```python
from build123d import *

# Parameters (mm, degrees)
BOSS_EXTRUDE1_DEPTH = 20
BOSS_EXTRUDE2_DEPTH = 20
SKETCH4_R           = 5
CUT_EXTRUDE1_DEPTH  = 2
SKETCH5_R           = 7
CUT_EXTRUDE2_DEPTH  = 2
BOSS_EXTRUDE5_DEPTH = 5
BOSS_EXTRUDE6_DEPTH = 2
SKETCH11_W          = 20
SKETCH11_H          = 5
SKETCH12_W          = 5
SKETCH12_H          = 5
BOSS_EXTRUDE7_DEPTH = 5
SKETCH13_R          = 1.5
BOSS_EXTRUDE8_DEPTH = 5
FILLET1_R           = 2.5


with BuildPart() as part:
    # Sketch2 → Boss-Extrude1 (new body)
    with BuildSketch(Plane(origin=(0, 0, 0), x_dir=(0, 0, -1), z_dir=(1, 0, 0))):
        with BuildLine():
            Line((-50, 0), (-45, 0))
            ThreePointArc((-45, 0), (0, 45), (45, 0))
            Line((45, 0), (50, 0))
            ThreePointArc((50, 0), (0, 50), (-50, 0))
        make_face()
    extrude(amount=BOSS_EXTRUDE1_DEPTH)

    # Sketch3 → Boss-Extrude2 (add)
    with BuildSketch(Plane(origin=(0, 0, 0), x_dir=(0, 0, -1), z_dir=(1, 0, 0))):
        Polygon((0, 45), (8, 45), (8, 50), (-8, 50), (-8, 45), align=None)
    extrude(amount=BOSS_EXTRUDE2_DEPTH)

    # Sketch4 → Cut-Extrude1 (cut)
    with BuildSketch(Plane(origin=(0, 50, 0), x_dir=(1, 0, 0), z_dir=(0, 1, 0))):
        with Locations(Location((10, 0, 0), (0, 0, 270))):
            Circle(SKETCH4_R)
    extrude(amount=-CUT_EXTRUDE1_DEPTH, mode=Mode.SUBTRACT)

    # Sketch5 → Cut-Extrude2 (cut)
    with BuildSketch(Plane(origin=(0, 48, 0), x_dir=(1, 0, 0), z_dir=(0, 1, 0))):
        with Locations(Location((10, 0, 0), (0, 0, 270))):
            Circle(SKETCH5_R)
    extrude(amount=-CUT_EXTRUDE2_DEPTH, mode=Mode.SUBTRACT)

    # Sketch9 → Boss-Extrude5 (add)
    with BuildSketch(Plane.ZY):
        with BuildLine():
            Line((10, 46.946778377), (11.041666667, 51.837067792))
            ThreePointArc((11.041666667, 51.837067792), (5.551369518, 52.708465131), (0, 53))
            Line((0, 53), (0, 48))
            ThreePointArc((0, 48), (5.027655412, 47.735968421), (10, 46.946778377))
        make_face()
    extrude(amount=BOSS_EXTRUDE5_DEPTH)

    # Sketch10 → Boss-Extrude6 (add)
    with BuildSketch(Plane.ZY.offset(5)):
        with BuildLine():
            Line((10, 46.946778377), (11.666666667, 54.77124144))
            ThreePointArc((11.666666667, 54.77124144), (5.865597981, 55.691963157), (0, 56))
            Line((0, 56), (0, 48))
            ThreePointArc((0, 48), (5.027655412, 47.735968421), (10, 46.946778377))
        make_face()
    extrude(amount=BOSS_EXTRUDE6_DEPTH)

    # Cut-Sweep2: sweep along a curve in space
    with BuildLine() as cut_sweep2_path:
        ThreePointArc((0, 48.902894143, 10.416666667), (0, 31.45764348, 38.864079388), (0, 0, 50))
    # Sketch11 → Cut-Sweep2 (sweep, cut)
    with BuildSketch(Plane.XZ):
        with Locations((10, 47.5)):
            Rectangle(SKETCH11_W, SKETCH11_H)
    sweep(path=cut_sweep2_path.line, mode=Mode.SUBTRACT)

    # Sketch12 → Boss-Extrude7 (add)
    with BuildSketch(Plane(origin=(0, 0, 0), x_dir=(1, 0, 0), z_dir=(0, -0.20833333333333337, 0.9780578828587918))):
        with Locations((7.5, 47.5)):
            Rectangle(SKETCH12_W, SKETCH12_H)
    boss_extrude7 = extrude(amount=BOSS_EXTRUDE7_DEPTH)

    # Sketch13 → Boss-Extrude8 (add, symmetric)
    with BuildSketch(Plane.ZY.offset(-5)):
        with Locations((14.786122748, 45.416082769)):
            Circle(SKETCH13_R)
    boss_extrude8 = extrude(amount=BOSS_EXTRUDE8_DEPTH, both=True)

    # Mirror1: Boss-Extrude7, Boss-Extrude8 across plane
    add(boss_extrude7.mirror(Plane(origin=(10, 42.970938062, 14.265289414), x_dir=(0, 0, 1), z_dir=(-1, 0, 0))))
    add(boss_extrude8.mirror(Plane(origin=(10, 42.970938062, 14.265289414), x_dir=(0, 0, 1), z_dir=(-1, 0, 0))))

    # Fillet1
    fillet1_edges = [part.edges().sort_by_distance(p)[0] for p in [
        (10, 0, -45),
        (20, 0, -47.5),
        (10, 0, -50),
        (0, 0, -47.5),
        (0, 34.977671449, -28.311879132),
        (20, 34.977671449, -28.311879132),
    ]]
    fillet(fillet1_edges, radius=FILLET1_R - 0.0001)  # a hair under: the kernel refuses the full size


solid = part.part
```
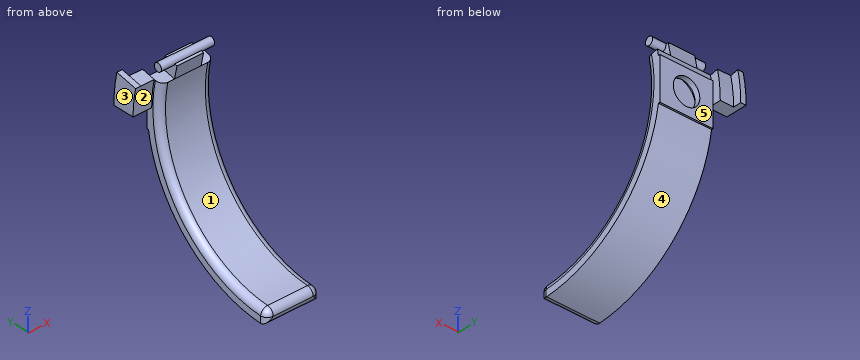
CAD build for the part. Positions are in the model's coordinates, mm. Face numbers are marked on the shaded views. A direction names the side the tool comes from. Round coordinates to 2 decimals unless told otherwise and drop trailing zeros. Loops run counter-clockwise (first coordinate to the right, second up) from the corner with the lowest first, then second, coordinate; pieces in that order, holes last. Notation, with made-up numbers: M 55.5,18 L 83.5,18 A22 cw 83.5,53 Z; hole C -34.75,42 d1. An arc over 180 degrees is marked long. Use a Markdown table: item, result. Add a question column.
(1) Which spindle directions (+Z, -Z, +X, -X, +Y, -Y) get a long thin tool onto all of the face, cutting with end or side? Do the marked faces 4 and 5. Say none if no direction does.
(2) Drill centre lines: line 1 (X direction, y = 47.25, z = 0); line 2 (Y direction, x = 14.25, z = -0.5); line 3 (Y direction, x = 5, z = -4). Where is each one in solid material? Low to high.
(3) Flat gauge pins, fed straight in: pin 1 (2 mm diameter, centred on x = -4.5, y = 52, fed in from -Z); pin 2 (10 mm diameter, centred on x = 8.5, y = 44, fed in from +Z); pin 3 (14.5 mm diameter, centred on y = 18.5, z = -34, fed in from -X); pin 4 (8 mm diameter, centred on x = 1.5, y = 38, fed in from -Z). Where does each tip first touch, or does it go through?
(4) Cut at B-B (x = 1.5). Give the cut face in (y, z), and give its area (3 significant figures).
(5) Pull direction Z, two halves, no side cores. Call the marked faces 1, 2 and 3: +Z half, -Z half, draft (parallel to the pull), parting line (faces both ways), or undercut.
Geometry says:
| question | item | result |
|---|---|---|
| 1 | face 4 | -Z, +X, -X, +Y |
| 1 | face 5 | +Z, -Z, +X, +Y |
| 2 | line 1 | x = 0.01 to 3, 17 to 19.99 |
| 2 | line 2 | y = 45 to 46 |
| 2 | line 3 | y = 44.82 to 46, 48 to 50 |
| 3 | pin 1 | stops at z = 0 |
| 3 | pin 2 | stops at z = 16.29 |
| 3 | pin 3 | stops at x = 0.53 |
| 3 | pin 4 | stops at z = -36.66 |
| 4 | outline | M 0.21,-48.43 A2.5 ccw 2.63,-49.93 A50 ccw 49.36,-8 L 50,-8 L 50,8 L 49.36,8 A50 ccw 48.9,10.42 L 44.22,9.42 A45.21 cw 2.38,-45.15 A2.29 ccw 0.21,-47.43 Z; C 45.42,14.79 d3 |
| 4 | area | 414 mm² |
| 5 | face 1 | undercut |
| 5 | face 2 | -Z half |
| 5 | face 3 | draft |
